```python
from build123d import *

# Parameters (mm, degrees)
FILLET1_R = 8
FILLET2_R = 1


with BuildPart() as part:
    # Sketch2 → Revolve2 (revolve)
    with BuildSketch(Plane.XY, mode=Mode.PRIVATE) as revolve2_sk:
        Polygon((50, 0), (70, 0), (70, 20), (50, 20), (33, 145), (35, 145), (35, 185), (25, 185), (25, 129.61723322), (42.219943718, 3), (50, 3), align=None)
    revolve(revolve2_sk.sketch.rotate(Axis((0, 0, 0), (0, 1, 0)), 90), axis=Axis((0, 0, 0), (0, 1, 0)))

    # Fillet1
    fillet1_edges = [part.edges().sort_by_distance(p)[0] for p in [
        (0, 20, 50),
    ]]
    fillet(fillet1_edges, radius=FILLET1_R)

    # Fillet2
    fillet2_edges = [part.edges().sort_by_distance(p)[0] for p in [
        (0, 145, 33),
    ]]
    fillet(fillet2_edges, radius=FILLET2_R)


solid = part.part
```
Check sheet for the modelled part. Datum: model origin and axes. Units: mm. A direction names the side the tool comes from. Coordinates: 2 decimals unless noted, no trailing zeros. Loops run counter-clockwise (first coordinate to the right, second up) from the corner with the lowest first, then second, coordinate; pieces in that order, holes last. Notation, with made-up numbers: M 20.5,30.5 L 67.5,30.5 A19 cw 67.5,63.5 Z; hole C 8.25,28 d4. An arc over 180 degrees is marked long. Answer as a JSON object with one key per item and string values.
1. Access from +Z, -Z, +X, -X, +Y, -Y to the whole of each face (thin tool, end or side, straight path). Record for faces 1 (the cylindrical face through (68.335, 10.14, 15.175)), 2 (the cylindrical face through (-15.02, 1.48, -47.69)), 3 (the cylindrical face through (34.168, 165.28, 7.587)).
Outcome:
{"face 1": "+Y, -Y", "face 2": "-Y", "face 3": "+Y"}
2. Release check for a two-part mould opening along Z. For faces 4 (the conical face through (36.37, 86.21, -18.92)), 5 (the flat face through (7.6, 145, 33.5)), 6 (the conical face through (29.925, 65.422, -15.565)) record: pulls with the +Z half, pulls with the -Z half, needs draft (parallel to the pull), parting line crosses it, or undercut.
Outcome:
{"face 4": "parting line crosses it", "face 5": "needs draft", "face 6": "undercut"}
3. Depth check by flat-ended pin: P1, Ø1, axis at x = 40.5, y = 55.5, coming from the +Z side; P2, Ø3, axis at y = 119, z = 13, coming from the +X side; P3, Ø6, axis at y = 90, z = 38.5, coming from the -X side; P4, Ø12, axis at x = -1.5, z = -23.5, coming from the +Y side. Enter the tip coordinate at first touch or a pass-through.
Outcome:
{"P1": "z = 21", "P2": "x = 34.72", "P3": "x = -19.52", "P4": "y = 185"}
4. Sectioned sample at A-A on x = 0. Record the cut outline in (y, z).
Outcome:
{"outline": "M 0,-70 L 20,-70 L 20,-56.99 A8 cw 26.92,-49.06 L 143.87,-33.15 A1 cw 145,-34.15 L 145,-35 L 185,-35 L 185,-25 L 129.62,-25 L 3,-42.22 L 3,-50 L 0,-50 Z; M 0,50 L 3,50 L 3,42.22 L 129.62,25 L 185,25 L 185,35 L 145,35 L 145,34.15 A1 cw 143.87,33.15 L 26.92,49.06 A8 cw 20,56.99 L 20,70 L 0,70 Z"}
5. Sectioned sample at C-C on y = 42. Record the cut outline in (x, z).
Outcome:
{"outline": "C 0,0 d94.02; hole C 0,0 d73.83"}
6. Sectioned sample at B-B on z = 0. Record the cut outline in (x, y).
Outcome:
{"outline": "M -70,0 L -50,0 L -50,3 L -42.22,3 L -25,129.62 L -25,185 L -35,185 L -35,145 L -34.15,145 A1 cw -33.15,143.87 L -49.06,26.92 A8 cw -56.99,20 L -70,20 Z; M 25,129.62 L 42.22,3 L 50,3 L 50,0 L 70,0 L 70,20 L 56.99,20 A8 cw 49.06,26.92 L 33.15,143.87 A1 cw 34.15,145 L 35,145 L 35,185 L 25,185 Z"}
7. Sectioned sample at D-D on y = 162.5. Record the cut outline in (x, z), and give its area (3 significant figures).
Outcome:
{"outline": "C 0,0 d70; hole C 0,0 d50", "area": "1,880 mm²"}
8. Scan lines: L1, parallel to X at y = 146, z = 0; L2, parallel to X at y = 1, z = 0; L3, parallel to Y at x = 59.5, z = 5. Record each from-to range of solid material in increasing order. Write a range as from..to.
Outcome:
{"L1": "-35..-25, 25..35", "L2": "-70..-50, 50..70", "L3": "0..20"}
